Work out the finished part from the listing and answer in its coordinate system (mm). A direction names the side the tool comes from. Round coordinates to 2 decimals unless told otherwise and drop trailing zeros. Loops run counter-clockwise (first coordinate to the right, second up) from the corner with the lowest first, then second, coordinate; pieces in that order, holes last. Notation, with made-up numbers: (5.25, -24) - (33.25, -24) arc R17 ccw to (33.25, -19) - close; hole circle Ø6 at (27.25, 10). An arc over 180 degrees is marked (long way). Return JSON: item names as keys, results as strings.
from build123d import *

# Parameters (mm, degrees)
F1_DEPTH = 15
F3_START = -45
F2_R     = 1.5
F3_DEPTH = 10
F4_W     = 4
F4_H     = 13
F5_DEPTH = 30
F6_W     = 5
F6_H     = 10
F7_DEPTH = 18.5400284665
F8_R     = 1


with BuildPart() as f1:
    # F0 (on Front) → F1 (new body)
    with BuildSketch(Plane.XZ):
        Polygon((13.3974596216, 50), (0, 0), (6.2116570825, 0), (19.1930145793, 48.4470857294), align=None)
    extrude(amount=F1_DEPTH)

    # F2 (on face) → F3 (cut)
    with BuildSketch(Plane(origin=(13.3974596216, 0, 50), x_dir=(0.9659258263, 0, -0.2588190451), z_dir=(0.2588190451, 0, 0.9659258263)).offset(F3_START)):
        with Locations((3, -12.5)):
            Circle(F2_R)
        with Locations((3, -2.5)):
            Circle(F2_R)
    extrude(amount=-F3_DEPTH, mode=Mode.SUBTRACT)

    # F4 (on face) → F5 (cut)
    with BuildSketch(Plane(origin=(13.3974596216, 0, 50), x_dir=(0.9659258263, 0, -0.2588190451), z_dir=(0.2588190451, 0, 0.9659258263))):
        with Locations((3, -7.5)):
            Rectangle(F4_W, F4_H)
    extrude(amount=-F5_DEPTH, mode=Mode.SUBTRACT)

    # F6 (on face) → F7 (cut, through all)
    with BuildSketch(Plane(origin=(0, 0, 0), x_dir=(0, -1, 0), z_dir=(-0.9659258263, 0, 0.2588190451))):
        with Locations((7.5, 15)):
            Rectangle(F6_W, F6_H)
    extrude(amount=-F7_DEPTH, mode=Mode.SUBTRACT)

    # F8
    f8_edges = [f1.edges().sort_by_distance(p)[0] for p in [
        (10.4811, -1, 35.252294),
        (14.344803, -14, 34.217017),
        (10.4811, -14, 35.252294),
        (14.344803, -1, 34.217017),
    ]]
    fillet(f8_edges, radius=F8_R)


solid = f1.part
1) Determine the mould class of faces 1 (the flat face through (10, -15, 25)), 2 (the flat face through (6.793, -7.395, 25.35)), 3 (the flat face through (8.504, -7.409, 20.253)) for opening direction Z: pulls with the +Z half, pulls with the -Z half, needs draft (parallel to the pull), parting line crosses it, or undercut.
Verdict:
{"face 1": "needs draft", "face 2": "pulls with the +Z half", "face 3": "undercut"}
2) A tool of negligible diameter and unlimited length cuts with its end or side. For faces 4 (the flat face through (10.535, -7.577, 35.455)), 5 (the flat face through (10, 0, 25)), 6 (the flat face through (8.034, -7.465, 18.553)), from which of +Z, -Z, +X, -X, +Y, -Y can it reach the whole face along a straight path? Write none if from no direction.
Verdict:
{"face 4": "none", "face 5": "+Z, -Z, +X, -X, +Y", "face 6": "-X"}
3) Find the intervals of material crossed by L1, parallel to X at y = -3, z = 22; L2, parallel to X at y = -5.75, z = 36; L3, parallel to X at y = -12.5, z = 13.5, in increasing order.
Verdict:
{"L1": "x = 5.89 to 6.93, 11.07 to 12.11", "L2": "x = 9.65 to 10.68, 14.82 to 15.86", "L3": "x = 3.62 to 9.83"}
4) Section B-B (z = 14) is taken. Give the vertices of the cut face in (x, y), and give its area (3 significant figures).
Verdict:
{"outline": "(3.75, -15) - (9.96, -15) - (9.96, -10) - (3.75, -10) - close; (3.75, -5) - (9.96, -5) - (9.96, 0) - (3.75, 0) - close", "area": "62.1 mm2"}
5) A flat-ended cylindrical pin translates along its axis: pin 1 (2 mm diameter, centred on x = 4, y = -8, fed in from +Z). Find the tip coordinate at first contact, or state that the pin passes through.
Verdict:
{"pin 1": "stops at z = 9.55"}
6) Section D-D (z = 4) is taken. Count the separate pieces of the cut face and the enclosed holes in it, and give its area (3 significant figures).
Verdict:
{"separate pieces": "1", "enclosed holes": "2", "area": "78.5 mm2"}
7) Section A-A (y = -9) is taken. Give the vertices of the cut face in (x, z).
Verdict:
{"outline": "(0, 0) - (6.21, 0) - (8.38, 8.11) - (2.59, 9.66) - close; (5.18, 19.32) - (10.97, 17.77) - (19.19, 48.45) - (18.23, 48.71) - (10.46, 19.73) - (6.6, 20.76) - (14.36, 49.74) - (13.4, 50) - close"}
8) Section C-C (y = -13.5) is taken. Give the vertices of the cut face in (x, z).
Verdict:
{"outline": "(0, 0) - (1.95, 0) - (3.57, 6.05) - (5.73, 5.47) - (4.26, 0) - (6.21, 0) - (19.19, 48.45) - (18.1, 48.74) - (10.33, 19.76) - (6.73, 20.73) - (14.49, 49.71) - (13.4, 50) - close"}
